Geometry check sheet. Reference: drawing and pictorial views, mm from the part's lowest x, y, z. Round coordinates to 2 decimals unless told otherwise and drop trailing zeros. Order: outer loops, then holes, each group sorted by start corner. A loop starts at its lowest first (then second) coordinate and runs counter-clockwise, first axis right, second up.
(1) Sectioned sample at B-B, the plane z = 150. Enter the section's corners in (x, y).
(2) Sectioned sample at A-A, the plane x = 25. Enter the section's corners in (y, z).
(3) Thickness scan on probe 1 along Z at (x, y) = (40, 3.15); probe 2 along Z at (x, y) = (25, 2.1); probe 3 along X at (y, z) = (2.95, 280). Record the ranges inside material, lowest first.
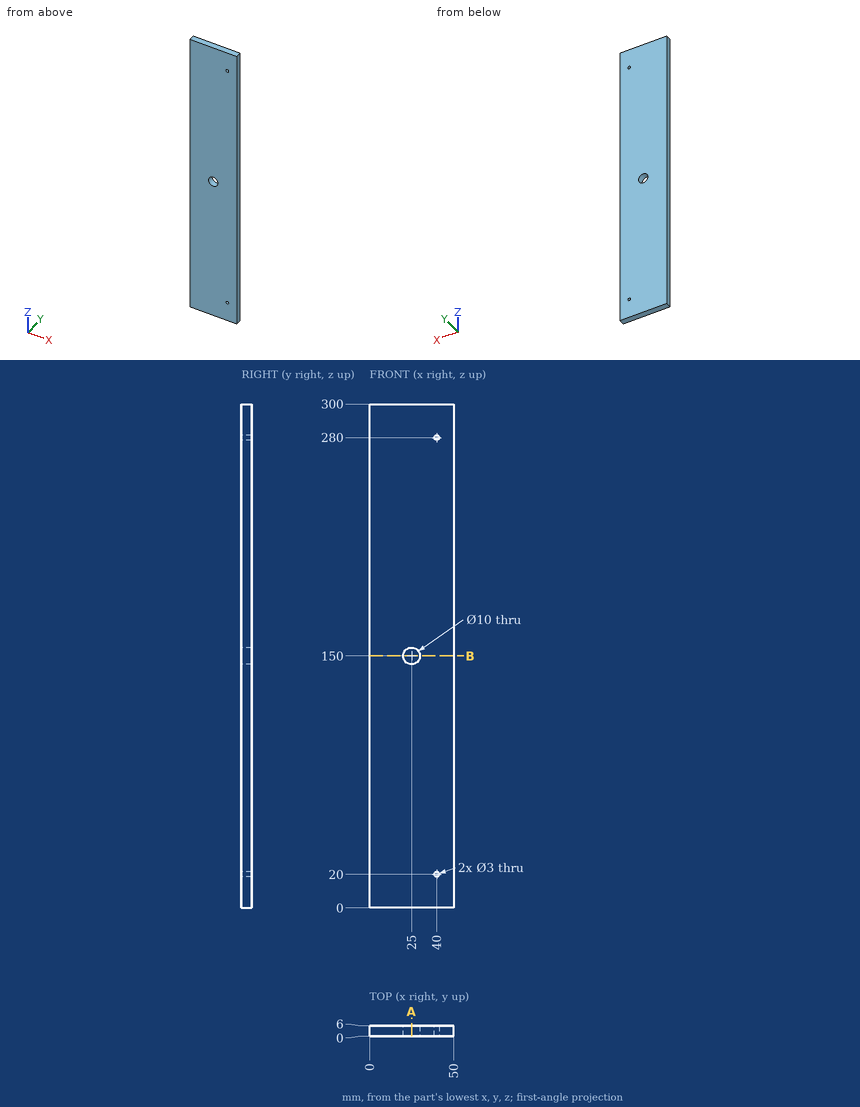
Derived:
1. outline: (0, 0) - (20, 0) - (20, 6) - (0, 6) - close; (30, 0) - (50, 0) - (50, 6) - (30, 6) - close
2. outline: (0, 0) - (6, 0) - (6, 145) - (0, 145) - close; (0, 155) - (6, 155) - (6, 300) - (0, 300) - close
3. probe 1: z = 0 to 18.5, 21.5 to 278.5, 281.5 to 300
3. probe 2: z = 0 to 145, 155 to 300
3. probe 3: x = 0 to 38.5, 41.5 to 50
